from build123d import *

# Parameters (mm, degrees)
ESQUISSE1_R        = 0.5
ESQUISSE1_R_2      = 1.5
ESQUISSE1_R_3      = 3.5
BOSS_EXTRU_1_DEPTH = 5


with BuildPart() as part:
    # Esquisse1 → Boss.-Extru.1 (new body)
    with BuildSketch(Plane.XY):
        with BuildLine():
            Line((0, 8), (20, 8))
            Line((20, 8), (27.728942549, 8))
            ThreePointArc((27.728942549, 8), (51.499017336, 0.032115491), (74.5, 10.0050005))
            ThreePointArc((74.5, 10.0050005), (81.783026213, 9.703645958), (81.02586797, 2.453818596))
            ThreePointArc((81.02586797, 2.453818596), (66.369841222, -5.316304031), (50, -8))
            Line((50, -8), (0, -8))
            Line((0, -8), (-15, -8))
            ThreePointArc((-15, -8), (-23, 0), (-15, 8))
            Line((-15, 8), (0, 8))
        make_face()
        with Locations((77.084290067, 5.654211565)):
            Circle(ESQUISSE1_R, mode=Mode.SUBTRACT)
        with Locations((15, 0)):
            Circle(ESQUISSE1_R_2, mode=Mode.SUBTRACT)
        with Locations((-15, 0)):
            Circle(ESQUISSE1_R_2, mode=Mode.SUBTRACT)
        Circle(ESQUISSE1_R_3, mode=Mode.SUBTRACT)
        with Locations((72.136277137, 1.439099698)):
            Circle(ESQUISSE1_R, mode=Mode.SUBTRACT)
    extrude(amount=BOSS_EXTRU_1_DEPTH)


solid = part.part
For this review, take the finished solid that the model builds, in its own axes (mm). Coordinates: 2 decimals unless noted, no trailing zeros. Loops run counter-clockwise (first coordinate to the right, second up) from the corner with the lowest first, then second, coordinate; pieces in that order, holes last. Notation, with made-up numbers: (-36, 52.25) - (3, 52.25) arc R21 ccw to (3, 66.25) - close; hole circle Ø10 at (-0.5, -27). An arc over 180 degrees is marked (long way). Use a Markdown table: item, result. Add a question column.
Item 1: For line 1 (Y direction, x = -15, z = 3.1); line 2 (Y direction, x = 14, z = 2); line 3 (Y direction, x = 24, z = 1.9), list the stretches that pass through material, from the lowest coordinate up.
Item 2: Insertion check: pin 1 Ø2.5 at (x, z) = (14, 3.5) entering from +Y; pin 2 Ø1 at (y, z) = (5, 3) entering from -X. Each pin has a flat end and moves straight along its axis. Give the tip position at first contact, or say it passes through.
Item 3: We need section D-D (y = -5.5). Give the boundary of the cut face in (x, z), and give its area (3 significant figures).
Item 4: We need section B-B (x = 15). Give the boundary of the cut face in (y, z).
Item 5: We need section A-A (x = 0). Give the boundary of the cut face in (y, z), and give its area (3 significant figures).
Item 6: Mouldability with a two-part tool opening along Y and no side actions: class faces 1 (the face through (6, 8, 2)), 2 (the face through (13.5, 0.07, 2.46)), 3 (the face through (-23, 0, 2)) as pulls with the +Y half, pulls with the -Y half, needs draft (parallel to the pull), parting line crosses it, or undercut.
Item 7: We need section C-C (z = 3.35). Give the boundary of the cut face in (x, y) (3 decimals).
Results list:
| question | item | result |
|---|---|---|
| 1 | line 1 | y = -8 to -1.5, 1.5 to 8 |
| 1 | line 2 | y = -8 to -1.12, 1.12 to 8 |
| 1 | line 3 | y = -8 to 8 |
| 2 | pin 1 | stops at y = 8 |
| 2 | pin 2 | stops at x = -21.61 |
| 3 | outline | (-20.81, 0) - (65.81, 0) - (65.81, 5) - (-20.81, 5) - close |
| 3 | area | 433 mm^2 |
| 4 | outline | (-8, 0) - (-1.5, 0) - (-1.5, 5) - (-8, 5) - close; (1.5, 0) - (8, 0) - (8, 5) - (1.5, 5) - close |
| 5 | outline | (-8, 0) - (-3.5, 0) - (-3.5, 5) - (-8, 5) - close; (3.5, 0) - (8, 0) - (8, 5) - (3.5, 5) - close |
| 5 | area | 45.0 mm^2 |
| 6 | face 1 | pulls with the +Y half |
| 6 | face 2 | undercut |
| 6 | face 3 | parting line crosses it |
| 7 | outline | (-15, -8) - (50, -8) arc R51.268 ccw to (81.026, 2.454) arc R5 ccw (long way) to (74.5, 10.005) arc R35 cw to (27.729, 8) - (-15, 8) arc R8 ccw to start; hole circle Ø3 at (-15, 0); hole circle Ø7 at (0, 0); hole circle Ø3 at (15, 0); hole circle Ø1 at (72.136, 1.439); hole circle Ø1 at (77.084, 5.654) |
